Verification items for the finished model (mm, model axes). Round coordinates to 2 decimals unless told otherwise and drop trailing zeros. Order: outer loops, then holes, each group sorted by start corner. A loop starts at its lowest first (then second) coordinate and runs counter-clockwise, first axis right, second up. Notation, with made-up numbers: M 61.25,66 L 71.25,66 A27 ccw 71.25,83 Z; hole C 60.25,-10.5 d8. An arc over 180 degrees is marked long. Answer as a JSON object with one key per item and string values. Group by question number.
```python
from build123d import *

# Parameters (mm, degrees)
SKETCH1_R           = 50.8
BOSS_EXTRUDE1_DEPTH = 6.6675
SKETCH2_R           = 20.2311
CUT_EXTRUDE1_DEPTH  = 74.06916056
SKETCH3_R           = 4.7625
CUT_EXTRUDE2_DEPTH  = 74.06916056
CIRPATTERN1_COUNT   = 6


with BuildPart() as part:
    # Sketch1 → Boss-Extrude1 (new, symmetric)
    with BuildSketch(Plane.XY):
        Circle(SKETCH1_R)
    extrude(amount=BOSS_EXTRUDE1_DEPTH, both=True)

    # Sketch2 → Cut-Extrude1 (cut, through all)
    with BuildSketch(Plane.XY.offset(6.6675)):
        Circle(SKETCH2_R)
    extrude(amount=-CUT_EXTRUDE1_DEPTH, mode=Mode.SUBTRACT)

    # Sketch3 → Cut-Extrude2 (cut, through all)
    with BuildSketch(Plane.XY.offset(6.6675)):
        with Locations((0, 42.8752)):
            Circle(SKETCH3_R)
    cut_extrude2 = extrude(amount=-CUT_EXTRUDE2_DEPTH, mode=Mode.SUBTRACT)

    # CirPattern1: Cut-Extrude2 ×6 about axis
    cirpattern1_axis = Axis((0, 0, 0), (0, 0, 1))
    for i in range(1, CIRPATTERN1_COUNT):
        add(cut_extrude2.rotate(cirpattern1_axis, i * 360 / CIRPATTERN1_COUNT), mode=Mode.SUBTRACT)


solid = part.part
```
Q1. Cross-section at A-A, the plane y = 0. Record the cut outline in (x, z).
Q2. Thickness scan on line 1 (Y direction, x = 0, z = 0.5); line 2 (X direction, y = -23, z = 6.25); line 3 (X direction, y = 13, z = 0.5). Record the ranges inside material, lowest first. Write a range as from..to.
Q3. Cross-section at C-C, the plane z = -0.5. Record the cut outline in (x, y) (1 decimal), then the cut area to 3 significant figures.
Q4. Release check for a two-part mould opening along X. For faces 1 (the face through (-11.012, -49.592, 0.093)), 2 (the face through (-41.89, -21.23, 0.09)), 3 (the face through (-2.2, -38.65, 0.09)), 4 (the face through (22, 1, 6.668)) record: released by +X, released by -X, zero draft, split by the parting line, or undercut.
Q5. Gauge pin test, flat ends, axial feed: pin 1 Ø5 at (y, z) = (-30.5, -3) entering from +X; pin 2 Ø3 at (x, z) = (-23, 4) entering from -Y; pin 3 Ø5 at (y, z) = (-37, 5) entering from +X; pin 4 Ø12 at (x, y) = (7.5, 12.5) entering from -Z. Record the tip position at first contact, or that the pin passes through.
Q6. Cross-section at D-D, the plane y = -12. Record the cut outline in (x, z), then the cut area to 3 significant figures.
Q7. Cross-section at B-B, the plane x = 0. Record the cut outline in (y, z), then the cut area to 3 significant figures.
Conclusion:
{
 "1": {"outline": "M -50.8,-6.67 L -20.23,-6.67 L -20.23,6.67 L -50.8,6.67 Z; M 20.23,-6.67 L 50.8,-6.67 L 50.8,6.67 L 20.23,6.67 Z"},
 "2": {"line 1": "-50.8..-47.64, -38.11..-20.23, 20.23..38.11, 47.64..50.8", "line 2": "-45.3..-41.63, -32.63..32.63, 41.63..45.3", "line 3": "-49.11..-15.5, 15.5..49.11"},
 "3": {"outline": "C 0,0 d101.6; hole C -37.1,-21.4 d9.5; hole C -37.1,21.4 d9.5; hole C 0,0 d40.5; hole C 0,-42.9 d9.5; hole C 0,42.9 d9.5; hole C 37.1,-21.4 d9.5; hole C 37.1,21.4 d9.5", "area": "6,390 mm2"},
 "4": {"face 1": "split by the parting line", "face 2": "undercut", "face 3": "undercut", "face 4": "zero draft"},
 "5": {"pin 1": "x = 42.39", "pin 2": "y = -46.03", "pin 3": "x = 37.29", "pin 4": "z = -6.67"},
 "6": {"outline": "M -49.36,-6.67 L -16.29,-6.67 L -16.29,6.67 L -49.36,6.67 Z; M 16.29,-6.67 L 49.36,-6.67 L 49.36,6.67 L 16.29,6.67 Z", "area": "882 mm2"},
 "7": {"outline": "M -50.8,-6.67 L -47.64,-6.67 L -47.64,6.67 L -50.8,6.67 Z; M -38.11,-6.67 L -20.23,-6.67 L -20.23,6.67 L -38.11,6.67 Z; M 20.23,-6.67 L 38.11,-6.67 L 38.11,6.67 L 20.23,6.67 Z; M 47.64,-6.67 L 50.8,-6.67 L 50.8,6.67 L 47.64,6.67 Z", "area": "561 mm2"}
}
